from build123d import *

# Parameters (mm, degrees)
BOSS_EXTRUDE3_DEPTH = 10


with BuildPart() as part:
    # Sketch5 → Boss-Extrude3 (new body)
    with BuildSketch(Plane.XY):
        with BuildLine():
            Line((0, 0), (0, -17.5))
            ThreePointArc((0, -17.5), (-1.464466094, -21.035533906), (-5, -22.5))
            Line((-5, -22.5), (-15, -22.5))
            Line((-15, -22.5), (-15, -20))
            Line((-15, -20), (-5, -20))
            ThreePointArc((-5, -20), (-3.232233047, -19.267766953), (-2.5, -17.5))
            Line((-2.5, -17.5), (-2.5, -0.001325618))
            ThreePointArc((-2.5, -0.001325618), (22.5, 25.024519835), (47.5, -0.001325618))
            Line((47.5, -0.001325618), (47.5, -17.5))
            ThreePointArc((47.5, -17.5), (48.232233047, -19.267766953), (50, -20))
            Line((50, -20), (60, -20))
            Line((60, -20), (60, -22.5))
            Line((60, -22.5), (50, -22.5))
            ThreePointArc((50, -22.5), (46.464466094, -21.035533906), (45, -17.5))
            Line((45, -17.5), (45, 0))
            ThreePointArc((45, 0), (22.5, 22.524519835), (0, 0))
        make_face()
    extrude(amount=BOSS_EXTRUDE3_DEPTH)


solid = part.part
The model under review builds one solid part; all positions refer to its coordinate system, in mm. A direction names the side the tool comes from. Round coordinates to 2 decimals unless told otherwise and drop trailing zeros. Loops run counter-clockwise (first coordinate to the right, second up) from the corner with the lowest first, then second, coordinate; pieces in that order, holes last. Notation, with made-up numbers: (9.5, 42) -> (14.5, 42) arc R24 cw to (14.5, 81) -> close; hole circle Ø8 at (86.5, 37.5). An arc over 180 degrees is marked (long way). Write item = value, one per line. Start each with the question number.
Item 1: Insertion check: pin 1 (10 mm diameter, centred on x = 35.5, y = -12.5, fed in from +Z); pin 2 (5 mm diameter, centred on y = -10.5, z = 3, fed in from -X); pin 3 (1 mm diameter, centred on y = 10, z = 7, fed in from -X); pin 4 (5 mm diameter, centred on x = 56.5, z = 5.5, fed in from +Y). Each pin has a flat end and moves straight along its axis. Give the tip position at first contact, or say it passes through.
Item 2: Take a section at C-C on y = 18.5. Give the boundary of the cut face in (x, z), plus the area to 3 significant figures.
Item 3: Mouldability with a two-part tool opening along Y and no side actions: class faces 6 (the flat face through (-10, -20, 5)), 7 (the flat face through (0, -9, 5)), 8 (the flat face through (-10, -22.5, 5)) as released by +Y, released by -Y, zero draft, split by the parting line, or undercut.
Item 4: Take a section at B-B on z = 9. Give the boundary of the cut face in (x, y).
Item 5: Take a section at D-D on x = 22.5. Give the boundary of the cut face in (y, z), plus the area to 3 significant figures.
Item 6: To check wall thickness, follow L1, parallel to X at y = -2, z = 8.75; L2, parallel to Y at x = -9, z = 0.5; L3, parallel to X at y = 11, z = 7.5. State the ranges of each line that lie inside material, in increasing order.
Item 7: Take a section at A-A on y = -11.5. Give the boundary of the cut face in (x, z), plus the area to 3 significant figures.
Item 8: For faces 1 (the flat face through (47.5, -9, 5)), 2 (the flat face through (60, -21, 5)), 3 (the flat face through (45, -9, 5)), 4 (the flat face through (3, 12, 10)), 5 (the flat face through (-2.5, -9, 5)), list the 3-axis set-ups (+Z, -Z, +X, -X, +Y, -Y) from which the entire face can be reached by the end or side of a thin tool; tool diameter is ignored.
Result:
q1.pin_1 = through
q1.pin_2 = -2.5
q1.pin_3 = -0.63
q1.pin_4 = -20
q2.outline = (5.66, 0) -> (9.66, 0) -> (9.66, 10) -> (5.66, 10) -> close; (35.34, 0) -> (39.34, 0) -> (39.34, 10) -> (35.34, 10) -> close
q2.area = 80.0 mm²
q3.face_6 = released by +Y
q3.face_7 = zero draft
q3.face_8 = released by -Y
q4.outline = (-15, -22.5) -> (-5, -22.5) arc R5 ccw to (0, -17.5) -> (0, 0) arc R22.5 cw to (45, 0) -> (45, -17.5) arc R5 ccw to (50, -22.5) -> (60, -22.5) -> (60, -20) -> (50, -20) arc R2.5 cw to (47.5, -17.5) -> (47.5, 0) arc R25 ccw to (-2.5, 0) -> (-2.5, -17.5) arc R2.5 cw to (-5, -20) -> (-15, -20) -> close
q5.outline = (22.52, 0) -> (25.02, 0) -> (25.02, 10) -> (22.52, 10) -> close
q5.area = 25.0 mm²
q6.L1 = -2.5 to 0, 45 to 47.5
q6.L2 = -22.5 to -20
q6.L3 = 0.04 to 2.86, 42.14 to 44.96
q7.outline = (-2.5, 0) -> (0, 0) -> (0, 10) -> (-2.5, 10) -> close; (45, 0) -> (47.5, 0) -> (47.5, 10) -> (45, 10) -> close
q7.area = 50.0 mm²
q8.face_1 = +Z, -Z, +X, +Y
q8.face_2 = +Z, -Z, +X, +Y, -Y
q8.face_3 = +Z, -Z, -Y
q8.face_4 = +Z, +X, -X, +Y, -Y
q8.face_5 = +Z, -Z, -X, +Y
